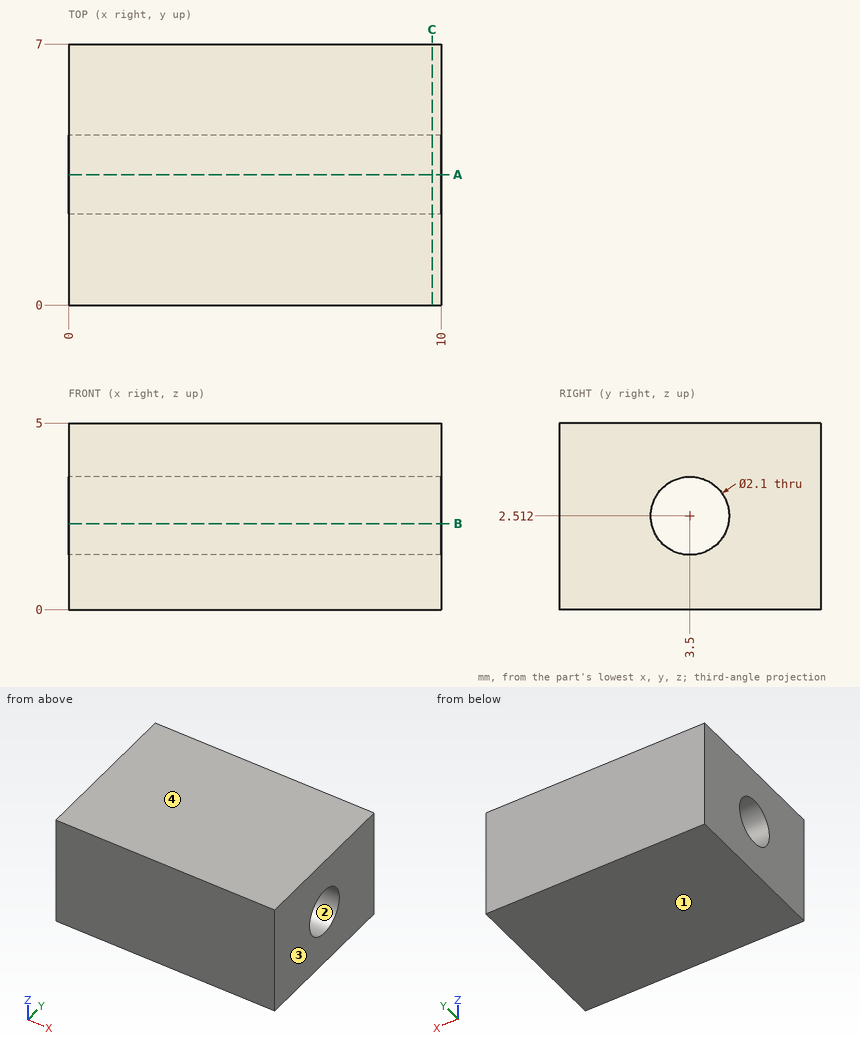
Geometry check sheet. Reference: drawing and pictorial views, mm from the part's lowest x, y, z. Give positions to 0.01 mm unless a question says otherwise; leave off trailing zeros. Order: outer loops, then holes, each group sorted by start corner. A loop starts at its lowest first (then second) coordinate and runs counter-clockwise, first axis right, second up. Notation, with made-up numbers: M 80.25,67.5 L 111.25,67.5 A29 ccw 111.25,97.5 Z; hole C 27.5,63 d3. An arc over 180 degrees is marked long. Answer as a JSON object with one key per item and string values. Group by question number.
1) Scan lines: line 1 along Z through (x, y) = (4.5, 3.5); line 2 along Y through (x, z) = (4, 2.5); line 3 along Z through (x, y) = (8, 3.25). Record each from-to range of solid material in increasing order. Write a range as [from, to].
2) Cross-section at C-C (x = 9.75). Enter the section's corners in (y, z).
3) Cross-section at A-A (y = 3.5). Enter the section's corners in (x, z), then the cut area to 3 significant figures.
4) Mould release check, pull along Z, two halves, no side actions. Record for the marked faces 1, 2, 3 and 4: released by +Z, released by -Z, zero draft, split by the parting line, or undercut.
5) Cross-section at B-B (z = 2.3). Enter the section's corners in (x, y), then the cut area to 3 significant figures.
Result sheet:
{
 "1": {"line 1": "z = [0, 1.46], [3.56, 5]", "line 2": "y = [0, 2.45], [4.55, 7]", "line 3": "z = [0, 1.49], [3.53, 5]"},
 "2": {"outline": "M 0,0 L 7,0 L 7,5 L 0,5 Z; hole C 3.5,2.51 d2.1"},
 "3": {"outline": "M 0,0 L 10,0 L 10,1.46 L 0,1.46 Z; M 0,3.56 L 10,3.56 L 10,5 L 0,5 Z", "area": "29.0 mm2"},
 "4": {"face 1": "released by -Z", "face 2": "undercut", "face 3": "zero draft", "face 4": "released by +Z"},
 "5": {"outline": "M 0,0 L 10,0 L 10,2.47 L 0,2.47 Z; M 0,4.53 L 10,4.53 L 10,7 L 0,7 Z", "area": "49.4 mm2"}
}
